Study the drawing (mm; zero at the part's minimum x, y, z) and answer. A direction names the side the tool comes from. Round coordinates to 2 decimals unless told otherwise and drop trailing zeros. Write each loop counter-clockwise with the first axis right and the second up, starting at its lowest first coordinate (ties: lowest second). Pieces come first, ordered by that corner, then holes. Notation, with made-up numbers: (14.25, 18) - (35.25, 18) arc R26 ccw to (35.25, 34) - close; hole circle Ø7 at (13.5, 18). An arc over 180 degrees is marked (long way). Use one line per item in the form item = value. Start each with the question number.
1) Each of these flat-tipped pins is pushed along its axis until it touches: pin 1 (5 mm diameter, centred on x = 23.5, y = 14.5, fed in from +Z); pin 2 (8 mm diameter, centred on x = 18.5, y = 23.5, fed in from -Z); pin 3 (6 mm diameter, centred on y = 26.5, z = 6.5, fed in from -X). Where does it stop, or does it pass through?
2) For a pull along Z with two mould halves and no side action, classify the marked faces 3, 4 and 5 as released by +Z, released by -Z, zero draft, split by the parting line, or undercut.
3) The part is cut by section B-B, the plane y = 17.75. Give the vertices of the cut face in (x, z).
4) For the marked faces 1 and 2, determine the directions among +Z, -Z, +X, -X, +Y, -Y from which every point of the face is accessible in a straight line to the end or side of a thin tool.
5) The part is cut by section A-A, the plane x = 20. Give the vertices of the cut face in (y, z).
6) Consider line 1 along Z through (x, y) = (20, 6.25); line 2 along Y through (x, z) = (19.5, 18); line 3 along Z through (x, y) = (17, 23.75). Determine where each line is inside the solid, lowest interval first. Write a range as from..to.
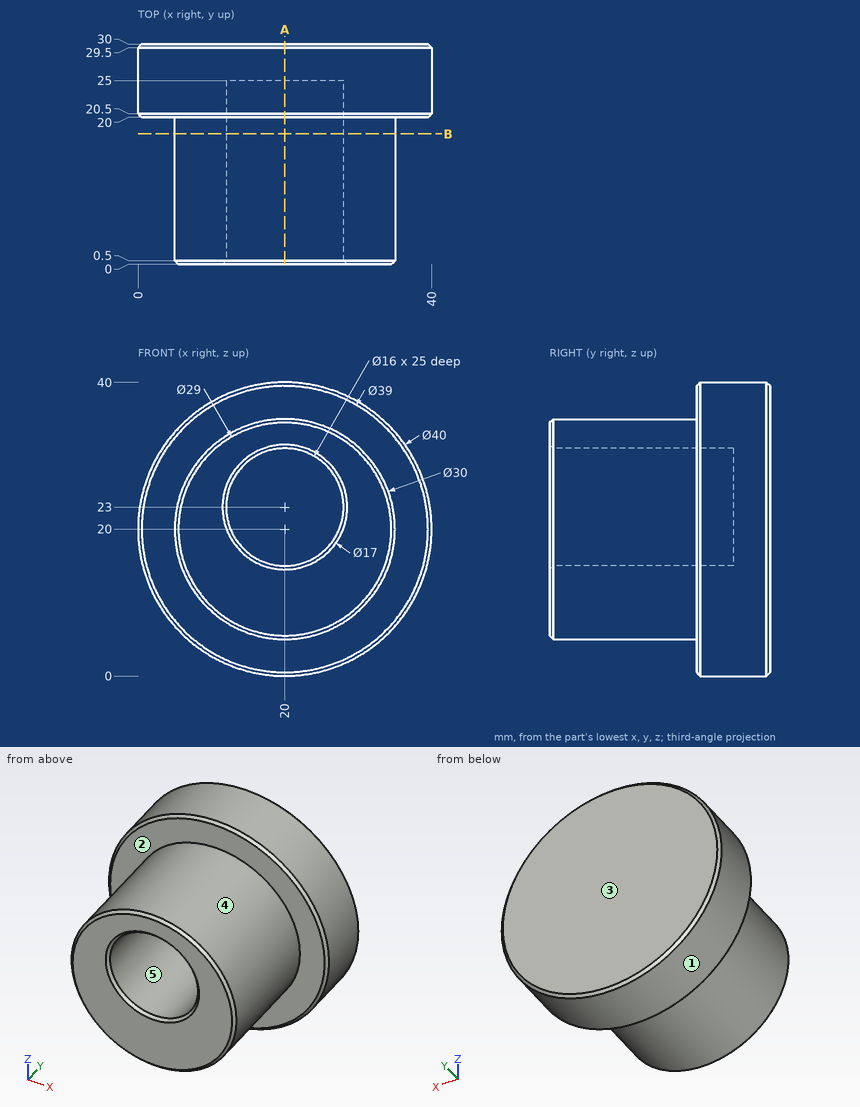
Geometry results:
q1.pin_1 = 34.97
q1.pin_2 = 0
q1.pin_3 = 2.98
q2.face_3 = zero draft
q2.face_4 = split by the parting line
q2.face_5 = undercut
q3.outline = circle Ø30 at (20, 20); hole circle Ø16 at (20, 23)
q4.face_1 = +Y, -Y
q4.face_2 = -Y
q5.outline = (0, 5.5) - (0.5, 5) - (20, 5) - (20, 0.5) - (20.5, 0) - (29.5, 0) - (30, 0.5) - (30, 39.5) - (29.5, 40) - (20.5, 40) - (20, 39.5) - (20, 35) - (0.5, 35) - (0, 34.5) - (0, 31.5) - (0.5, 31) - (25, 31) - (25, 15) - (0.5, 15) - (0, 14.5) - close
q6.line_1 = 5..15, 31..35
q6.line_2 = 25..30
q6.line_3 = 0.23..15.58, 30.42..39.77
